Here's the drawing with two shaded views (mm, measured from the low corner). I have some questions. A direction names the side the tool comes from. Round coordinates to 2 decimals unless told otherwise and drop trailing zeros. Order: outer loops, then holes, each group sorted by start corner. A loop starts at its lowest first (then second) coordinate and runs counter-clockwise, first axis right, second up. Notation, with made-up numbers: (82.5, 24) -> (127.5, 24) arc R22 cw to (127.5, 35) -> close; hole circle Ø6 at (-1.75, 72.5). An arc over 180 degrees is marked (long way). Answer in a Markdown table with one row per item.
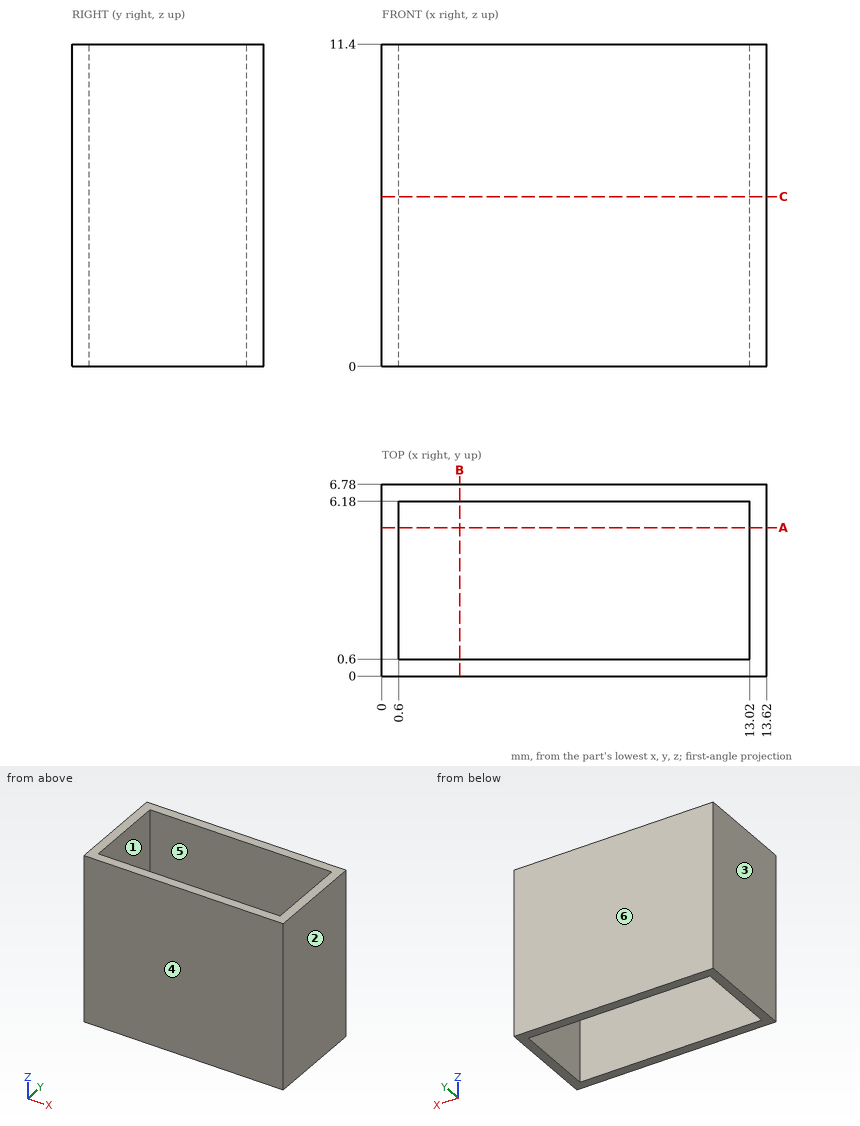
1. Suppose I cut it at C-C on z = 6. Write out the boundary of the cut face in (x, y).
Numbers:
| item | result |
|---|---|
| outline | (0, 0) -> (13.62, 0) -> (13.62, 6.78) -> (0, 6.78) -> close; hole (0.6, 0.6) -> (13.02, 0.6) -> (13.02, 6.18) -> (0.6, 6.18) -> close |
2. We'd pull the mould along Y, two halves only. Please class the marked faces 3, 4, 5 and 6: released by +Y, released by -Y, zero draft, split by the parting line, or undercut.
Numbers:
| item | result |
|---|---|
| face 3 | zero draft |
| face 4 | released by -Y |
| face 5 | undercut |
| face 6 | released by +Y |
3. Please list where these lines run through material, in increasing order: line 1 along X through (y, z) = (2, 1.25); line 2 along Y through (x, z) = (11.25, 7.5).
Numbers:
| item | result |
|---|---|
| line 1 | x = 0 to 0.6, 13.02 to 13.62 |
| line 2 | y = 0 to 0.6, 6.18 to 6.78 |
4. For the marked faces 1 and 2, which set-ups out of +Z, -Z, +X, -X, +Y, -Y let a thin tool reach every point of the face, with its end or its side?
Numbers:
| item | result |
|---|---|
| face 1 | +Z, -Z |
| face 2 | +Z, -Z, +X, +Y, -Y |
5. Suppose I cut it at B-B on x = 2.75. Write out the boundary of the cut face in (y, z), then the cut area to 3 significant figures.
Numbers:
| item | result |
|---|---|
| outline | (0, 0) -> (0.6, 0) -> (0.6, 11.4) -> (0, 11.4) -> close; (6.18, 0) -> (6.78, 0) -> (6.78, 11.4) -> (6.18, 11.4) -> close |
| area | 13.7 mm2 |
6. For pin 1 Ø1 at (x, y) = (4.5, 4.5) entering from +Z, with a flat end and sliding along its axis, tell me the tip position at first contact or that it passes through.
Numbers:
| item | result |
|---|---|
| pin 1 | passes through |
7. Suppose I cut it at A-A on y = 5.25. Write out the boundary of the cut face in (x, z).
Numbers:
| item | result |
|---|---|
| outline | (0, 0) -> (0.6, 0) -> (0.6, 11.4) -> (0, 11.4) -> close; (13.02, 0) -> (13.62, 0) -> (13.62, 11.4) -> (13.02, 11.4) -> close |
